```python
from build123d import *

# Parameters (mm, degrees)
F0_R     = 4
F1_DEPTH = 50
F2_R     = 6
F3_DEPTH = 4
F4_R     = 7
F5_DEPTH = 4


with BuildPart() as f1:
    # F0 (on Top) → F1 (new body, symmetric)
    with BuildSketch(Plane.XY):
        Circle(F0_R)
    extrude(amount=F1_DEPTH, both=True)

    # F2 (on face) → F3 (join)
    with BuildSketch(Plane.XY.offset(50)):
        Circle(F2_R)
    extrude(amount=-F3_DEPTH)

    # F4 (on face) → F5 (join)
    with BuildSketch(Plane(origin=(0, 0, -50), x_dir=(1, 0, 0), z_dir=(0, 0, -1))):
        Circle(F4_R)
    extrude(amount=-F5_DEPTH)


solid = f1.part
```
Check sheet for the modelled part. Datum: model origin and axes. Units: mm. A direction names the side the tool comes from. Give positions to 0.01 mm unless a question says otherwise; leave off trailing zeros. Write each loop counter-clockwise with the first axis right and the second up, starting at its lowest first coordinate (ties: lowest second). Pieces come first, ordered by that corner, then holes.
Item 1: Access from +Z, -Z, +X, -X, +Y, -Y to the whole of each face (thin tool, end or side, straight path). Record for faces 4 (the face through (-6, 0, 48)), 5 (the face through (-0.867, -3.905, 0.644)), 6 (the face through (0, 0, -50)).
Item 2: Cross-section at C-C (z = -2.5). Enter the section's corners in (x, y), and give its area (3 significant figures).
Item 3: Draft check along Z on faces 1 (the face through (0, 0, 50)), 2 (the face through (-1.42, -3.92, 46)), 3 (the face through (6.466, 2.681, -48.028)). Enter one of: released by +Z, released by -Z, zero draft, split by the parting line, or undercut.
Item 4: Gauge pin test, flat ends, axial feed: pin 1 (3 mm diameter, centred on x = 5, z = 28.5, fed in from +Y); pin 2 (5 mm diameter, centred on y = -1.5, z = -4.5, fed in from -X); pin 3 (1.5 mm diameter, centred on y = -2, z = -28.5, fed in from +X). Record the tip position at first contact, or that the pin passes through.
Item 5: Cross-section at A-A (x = 0). Enter the section's corners in (y, z).
Item 6: Scan lines: L1, parallel to Z at x = -4.5, y = -2.5; L2, parallel to Z at x = 2, y = -6.5; L3, parallel to Y at x = 0.5, z = 8. Record each from-to range of solid material in increasing order.
Report:
1. face 4: +Z
1. face 5: none
1. face 6: -Z, +X, -X, +Y, -Y
2. outline: circle Ø8 at (0, 0)
2. area: 50.3 mm2
3. face 1: released by +Z
3. face 2: undercut
3. face 3: zero draft
4. pin 1: stops at y = 1.94
4. pin 2: stops at x = -4
4. pin 3: stops at x = 3.8
5. outline: (-7, -50) - (7, -50) - (7, -46) - (4, -46) - (4, 46) - (6, 46) - (6, 50) - (-6, 50) - (-6, 46) - (-4, 46) - (-4, -46) - (-7, -46) - close
6. L1: z = -50 to -46, 46 to 50
6. L2: z = -50 to -46
6. L3: y = -3.97 to 3.97
